from build123d import *

# Parameters (mm, degrees)
SKETCH1_W           = 37.5
SKETCH1_H           = 22.5
BOSS_EXTRUDE2_DEPTH = 17.5
SKETCH2_R           = 0.625
BOSS_EXTRUDE3_DEPTH = 10
SKETCH3_R           = 8.75
BOSS_EXTRUDE4_DEPTH = 12.5
SKETCH4_R           = 8.25
BOSS_EXTRUDE5_DEPTH = 12.5
FILLET2_R           = 1.5
FILLET3_R           = 5
BOSS_EXTRUDE6_DEPTH = 10


with BuildPart() as part:
    # Sketch1 → Boss-Extrude2 (new body)
    with BuildSketch(Plane(origin=(0, 0, 0), x_dir=(0, 0, -1), z_dir=(1, 0, 0))):
        Rectangle(SKETCH1_W, SKETCH1_H)
    extrude(amount=BOSS_EXTRUDE2_DEPTH)

    # Sketch2 → Boss-Extrude3 (add)
    with BuildSketch(Plane(origin=(17.5, 0, 0), x_dir=(0, 0, -1), z_dir=(1, 0, 0))):
        with BuildLine():
            Line((10.915063509, 1.246479188), (6.584936491, 1.246479188))
            ThreePointArc((6.584936491, 1.246479188), (6.25, -0.003520812), (6.584936491, -1.253520812))
            Line((6.584936491, -1.253520812), (10.915063509, -1.253520812))
            ThreePointArc((10.915063509, -1.253520812), (11.25, -0.003520812), (10.915063509, 1.246479188))
        make_face()
        with Locations((8.75, -0.003520812)):
            Circle(SKETCH2_R, mode=Mode.SUBTRACT)
    extrude(amount=BOSS_EXTRUDE3_DEPTH)

    # Sketch3 → Boss-Extrude4 (add)
    with BuildSketch(Plane.XY.offset(18.75)):
        with Locations((8.75, 0)):
            Circle(SKETCH3_R)
    extrude(amount=BOSS_EXTRUDE4_DEPTH)

    # Sketch4 → Boss-Extrude5 (add)
    with BuildSketch(Plane.XY.offset(31.25)):
        with Locations((8.75, 0)):
            Circle(SKETCH4_R)
    extrude(amount=BOSS_EXTRUDE5_DEPTH)

    # Fillet2
    fillet2_edges = [part.edges().sort_by_distance(p)[0] for p in [
        (0.5, 0, 43.75),
    ]]
    fillet(fillet2_edges, radius=FILLET2_R)

    # Fillet3
    fillet3_edges = [part.edges().sort_by_distance(p)[0] for p in [
        (8.75, -11.25, -18.75),
        (8.75, 11.25, -18.75),
    ]]
    fillet(fillet3_edges, radius=FILLET3_R)

    # Sketch5 → Boss-Extrude6 (add)
    with BuildSketch(Plane.ZY):
        with BuildLine():
            ThreePointArc((-10.915063509, 1.25), (-11.164814566, 0.647047613), (-11.25, 0))
            Line((-11.25, 0), (-8.75, 0))
            Line((-8.75, 0), (-6.25, 0))
            ThreePointArc((-6.25, 0), (-6.335185434, 0.647047613), (-6.584936491, 1.25))
            Line((-6.584936491, 1.25), (-10.915063509, 1.25))
        make_face()
        with BuildLine():
            Line((-8.75, 0), (-11.25, 0))
            ThreePointArc((-11.25, 0), (-11.164814566, -0.647047613), (-10.915063509, -1.25))
            Line((-10.915063509, -1.25), (-6.584936491, -1.25))
            ThreePointArc((-6.584936491, -1.25), (-6.335185434, -0.647047613), (-6.25, 0))
            Line((-6.25, 0), (-8.75, 0))
        make_face()
    extrude(amount=BOSS_EXTRUDE6_DEPTH)


solid = part.part
Could you check a few things on this model? Use its own coordinates, in mm. A direction names the side the tool comes from. Round coordinates to 2 decimals unless told otherwise and drop trailing zeros. Write each loop counter-clockwise with the first axis right and the second up, starting at its lowest first coordinate (ties: lowest second). Pieces come first, ordered by that corner, then holes. Notation, with made-up numbers: (48, -28.5) -> (86, -28.5) arc R12 cw to (86, -21.5) -> close; hole circle Ø9 at (51.25, 5). An arc over 180 degrees is marked (long way). Use a Markdown table: item, result.
1. If we section it at A-A (z = -8.75): List the corners of the cut face in (x, y) for me.
Answer key:
| item | result |
|---|---|
| outline | (-10, -1.25) -> (0, -1.25) -> (0, -11.25) -> (17.5, -11.25) -> (17.5, -1.25) -> (27.5, -1.25) -> (27.5, -0.63) -> (17.5, -0.63) -> (17.5, 0.62) -> (27.5, 0.62) -> (27.5, 1.25) -> (17.5, 1.25) -> (17.5, 11.25) -> (0, 11.25) -> (0, 1.25) -> (-10, 1.25) -> close |
2. We'd pull the mould along Z, two halves only. Please class faces 4 (the face through (16.62, 2.48, 36.67)), 5 (the face through (22.43, -0.24, -9.33)), 6 (the face through (9, -9, 18.75)): +Z half, -Z half, draft (parallel to the pull), parting line (faces both ways), or undercut.
Answer key:
| item | result |
|---|---|
| face 4 | draft |
| face 5 | undercut |
| face 6 | +Z half |
3. Please list where these lines run through material, in increasing order: probe 1 along Y at (x, z) = (22, -8.75); probe 2 along Y at (x, z) = (24, -8); probe 3 along X at (y, z) = (9, 2).
Answer key:
| item | result |
|---|---|
| probe 1 | y = -1.25 to -0.63, 0.62 to 1.25 |
| probe 2 | y = -1.25 to 1.25 |
| probe 3 | x = 0 to 17.5 |
4. If we section it at B-B (x = 8.75): List the corners of the cut face in (y, z) for me, then the cut area to 3 significant figures.
Answer key:
| item | result |
|---|---|
| outline | (-11.25, -13.75) arc R5 ccw to (-6.25, -18.75) -> (6.25, -18.75) arc R5 ccw to (11.25, -13.75) -> (11.25, 18.75) -> (8.75, 18.75) -> (8.75, 31.25) -> (8.25, 31.25) -> (8.25, 42.25) arc R1.5 ccw to (6.75, 43.75) -> (-6.75, 43.75) arc R1.5 ccw to (-8.25, 42.25) -> (-8.25, 31.25) -> (-8.75, 31.25) -> (-8.75, 18.75) -> (-11.25, 18.75) -> close |
| area | 1,260 mm^2 |
5. If we section it at D-D (y = -10): List the corners of the cut face in (x, z) for me, then the cut area to 3 significant figures.
Answer key:
| item | result |
|---|---|
| outline | (0, -17.06) -> (17.5, -17.06) -> (17.5, 18.75) -> (0, 18.75) -> close |
| area | 627 mm^2 |
6. Which directions (+Z, -Z, +X, -X, +Y, -Y) give clear straight access to the entire face, cutting with the end or side of a thin tool? Please do faces 1 (the face through (-5, 1.25, -9)), 2 (the face through (17.5, 0, -9)), 3 (the face through (1.806, -5.324, 24.912)).
Answer key:
| item | result |
|---|---|
| face 1 | +Z, -Z, -X, +Y |
| face 2 | +X |
| face 3 | +Z |
7. For pin 1 Ø1.5 at (x, z) = (9.5, 29.5) entering from -Y; pin 2 Ø3.5 at (x, z) = (23, -9.5) entering from +Y; pin 3 Ø10 at (y, z) = (1.5, 15.5) entering from +X, each with a flat end and sliding along its axis, tell me the tip position at first contact or that it passes through.
Answer key:
| item | result |
|---|---|
| pin 1 | stops at y = -8.75 |
| pin 2 | stops at y = 1.25 |
| pin 3 | stops at x = 17.5 |
8. If we section it at C-C (x = 18.5): List the corners of the cut face in (y, z) for me (3 decimals).
Answer key:
| item | result |
|---|---|
| outline | (-1.254, -10.915) arc R2.5 ccw to (1.246, -10.915) -> (1.246, -6.585) arc R2.5 ccw to (-1.254, -6.585) -> close; hole circle Ø1.25 at (-0.004, -8.75) |
